The listing builds one solid part. Answer for the finished solid, in the listing's coordinates (mm). A direction names the side the tool comes from. Coordinates: 2 decimals unless noted, no trailing zeros. Loops run counter-clockwise (first coordinate to the right, second up) from the corner with the lowest first, then second, coordinate; pieces in that order, holes last. Notation, with made-up numbers: M -9,21 L 9,21 A6 cw 9,29 Z; hole C 41.5,89.25 d11. An arc over 180 degrees is marked long. Answer in a Markdown table with one row per item. Add a question column.
from build123d import *

# Parameters (mm, degrees)
SKETCH_1_W          = 166
SKETCH_1_H          = 70
EXTRUDE_1_DEPTH     = 3
SKETCH_2_W          = 3
SKETCH_2_H          = 20
CUT_EXTRUDE_1_DEPTH = 91.1276872
SKETCH_3_R          = 1.5
CUT_EXTRUDE_2_DEPTH = 91.1276872
SKETCH_4_R          = 1
CUT_EXTRUDE_3_DEPTH = 91.1276872
FILLET_1_R          = 1
SKETCH_5_R          = 22.5
CUT_EXTRUDE_4_DEPTH = 91.1276872
SKETCH_6_R          = 2.5
CUT_EXTRUDE_5_DEPTH = 91.1276872
FILLET_2_R          = 10
SKETCH_7_W          = 30
SKETCH_7_H          = 10
EXTRUDE_2_DEPTH     = 3
FILLET_START        = -1
FILLET_3_DEPTH      = 5
FILLET_3_2_DEPTH    = 3
SKETCH_8_R          = 1.5
CUT_EXTRUDE_6_DEPTH = 95.461632423
SKETCH_9_R          = 1.5
CUT_EXTRUDE_7_DEPTH = 95.461632423


with BuildPart() as part:
    # 草图1 → 凸台-拉伸1 (new body)
    with BuildSketch(Plane.XY):
        Rectangle(SKETCH_1_W, SKETCH_1_H)
    extrude(amount=EXTRUDE_1_DEPTH)

    # 草图2 → 切除-拉伸1 (cut, through all)
    with BuildSketch(Plane.XY.offset(3)):
        with Locations((-81.5, 0)):
            Rectangle(SKETCH_2_W, SKETCH_2_H)
    extrude(amount=-CUT_EXTRUDE_1_DEPTH, mode=Mode.SUBTRACT)

    # 草图3 → 切除-拉伸2 (cut, through all)
    with BuildSketch(Plane.XY.offset(3)):
        with Locations((-77, 27)):
            Circle(SKETCH_3_R)
        with Locations((-77, 17)):
            Circle(SKETCH_3_R)
        with Locations(Location((-77, -17, 0), (0, 0, 180))):
            Circle(SKETCH_3_R)
        with Locations(Location((-77, -27, 0), (0, 0, 180))):
            Circle(SKETCH_3_R)
    extrude(amount=-CUT_EXTRUDE_2_DEPTH, mode=Mode.SUBTRACT)

    # 草图4 → 切除-拉伸3 (cut, through all)
    with BuildSketch(Plane.XY.offset(3)):
        with Locations((-10, 22.6)):
            Circle(SKETCH_4_R)
        with Locations((8, 22.6)):
            Circle(SKETCH_4_R)
        with Locations(Location((8, -22.6, 0), (0, 0, 180))):
            Circle(SKETCH_4_R)
        with Locations(Location((-10, -22.6, 0), (0, 0, 180))):
            Circle(SKETCH_4_R)
    extrude(amount=-CUT_EXTRUDE_3_DEPTH, mode=Mode.SUBTRACT)

    # 圆角1
    fillet_1_edges = [part.edges().sort_by_distance(p)[0] for p in [
        (-83, -10, 1.5),
        (-83, 10, 1.5),
        (-83, -35, 1.5),
        (-83, 35, 1.5),
    ]]
    fillet(fillet_1_edges, radius=FILLET_1_R)

    # 草图5 → 切除-拉伸4 (cut, through all)
    with BuildSketch(Plane.XY.offset(3)):
        with Locations((38, 0)):
            Circle(SKETCH_5_R)
    extrude(amount=-CUT_EXTRUDE_4_DEPTH, mode=Mode.SUBTRACT)

    # 草图6 → 切除-拉伸5 (cut, through all)
    with BuildSketch(Plane.XY.offset(3)):
        with Locations((75, 27)):
            Circle(SKETCH_6_R)
        with Locations((-25, 27)):
            Circle(SKETCH_6_R)
        with Locations(Location((75, -27, 0), (0, 0, 180))):
            Circle(SKETCH_6_R)
        with Locations(Location((-25, -27, 0), (0, 0, 180))):
            Circle(SKETCH_6_R)
    extrude(amount=-CUT_EXTRUDE_5_DEPTH, mode=Mode.SUBTRACT)

    # 圆角2
    fillet_2_edges = [part.edges().sort_by_distance(p)[0] for p in [
        (83, -35, 1.5),
        (83, 35, 1.5),
    ]]
    fillet(fillet_2_edges, radius=FILLET_2_R)

    # 草图7 → 凸台-拉伸2 (add)
    with BuildSketch(Plane.XY.offset(3)):
        with Locations((28, 40)):
            Rectangle(SKETCH_7_W, SKETCH_7_H)
        with Locations((28, -40)):
            Rectangle(SKETCH_7_W, SKETCH_7_H)
    extrude(amount=-EXTRUDE_2_DEPTH)

    # 圆角3: read off the stored shape, not the designer's step
    # 圆角3 outline → 圆角3 (cut)
    with BuildSketch(Plane.XY.offset(FILLET_START)):
        with BuildLine():
            Line((13, -45), (18, -45))
            ThreePointArc((18, -45), (14.464466094, -43.535533906), (13, -40))
            Line((13, -40), (13, -45))
        make_face()
        with BuildLine():
            ThreePointArc((43, -40), (41.535533906, -43.535533906), (38, -45))
            Line((38, -45), (43, -45))
            Line((43, -45), (43, -40))
        make_face()
        with BuildLine():
            Line((43, 45), (38, 45))
            ThreePointArc((38, 45), (41.535533906, 43.535533906), (43, 40))
            Line((43, 40), (43, 45))
        make_face()
        with BuildLine():
            ThreePointArc((13, 40), (14.464466094, 43.535533906), (18, 45))
            Line((18, 45), (13, 45))
            Line((13, 45), (13, 40))
        make_face()
    extrude(amount=FILLET_3_DEPTH, mode=Mode.SUBTRACT)

    # Fillet 3 2 outline → Fillet 3 2 (add)
    with BuildSketch(Plane.XY):
        with BuildLine():
            Line((43, -35), (43, -40))
            ThreePointArc((43, -40), (44.464466094, -36.464466094), (48, -35))
            Line((48, -35), (43, -35))
        make_face()
        with BuildLine():
            ThreePointArc((8, -35), (11.535533906, -36.464466094), (13, -40))
            Line((13, -40), (13, -35))
            Line((13, -35), (8, -35))
        make_face()
        with BuildLine():
            Line((13, 35), (13, 40))
            ThreePointArc((13, 40), (11.535533906, 36.464466094), (8, 35))
            Line((8, 35), (13, 35))
        make_face()
        with BuildLine():
            ThreePointArc((48, 35), (44.464466094, 36.464466094), (43, 40))
            Line((43, 40), (43, 35))
            Line((43, 35), (48, 35))
        make_face()
    extrude(amount=FILLET_3_2_DEPTH)

    # 草图8 → 切除-拉伸6 (cut, through all)
    with BuildSketch(Plane(origin=(0, 0, 0), x_dir=(-1, 0, 0), z_dir=(0, 0, -1))):
        with Locations((-78, 0)):
            Circle(SKETCH_8_R)
    extrude(amount=-CUT_EXTRUDE_6_DEPTH, mode=Mode.SUBTRACT)

    # 草图9 → 切除-拉伸7 (cut, through all)
    with BuildSketch(Plane(origin=(0, 0, 0), x_dir=(-1, 0, 0), z_dir=(0, 0, -1))):
        with Locations((-29, 40)):
            Circle(SKETCH_9_R)
        with Locations(Location((-29, -40, 0), (0, 0, 180))):
            Circle(SKETCH_9_R)
    extrude(amount=-CUT_EXTRUDE_7_DEPTH, mode=Mode.SUBTRACT)


solid = part.part
(1) A cutting plane is placed at B-B (x = 20.5). Give the vertices of the cut face in (y, z), plus the area to 3 significant figures.
(2) A cutting plane is placed at D-D (x = 1). Give the vertices of the cut face in (y, z), plus the area to 3 significant figures.
(3) Each of these flat-tipped pins is pushed along its axis until it touches: pin 1 (3 mm diameter, centred on x = 75, y = 27, fed in from -Z); pin 2 (1.5 mm diameter, centred on y = -1, z = 2, fed in from -X); pin 3 (1.6 mm diameter, centred on x = -81, z = 1, fed in from -Y). Where does it stop, or does it pass through?
(4) Straight lines are drawn through the part: line 1 (Y direction, x = -77, z = 2.3); line 2 (X direction, y = -22.6, z = 1.6); line 3 (Y direction, x = -25, z = 2.3). For each, find the intervals that lie inside material, in ascending order.
(5) A cutting plane is placed at A-A (x = -25). Give the vertices of the cut face in (y, z).
(6) For faces 1 (the face through (-38, -35, 1)), 2 (the face through (-80, 0, 2)), 3 (the face through (-1, 1, 0)), 4 (the face through (-38, 35, 1)), 5 (the face through (27.8, -39.1, 1.5)), determine the directions among +Z, -Z, +X, -X, +Y, -Y from which every point of the face is accessible in a straight line to the end or side of a thin tool.
(7) A cutting plane is placed at C-C (z = 1.1). State how many separate pieces and enclosed holes the cut face has, plus the area to 3 significant figures.
Solved:
| question | item | result |
|---|---|---|
| 1 | outline | M -45,0 L -14.14,0 L -14.14,3 L -45,3 Z; M 14.14,0 L 45,0 L 45,3 L 14.14,3 Z |
| 1 | area | 185 mm² |
| 2 | outline | M -35,0 L 35,0 L 35,3 L -35,3 Z |
| 2 | area | 210 mm² |
| 3 | pin 1 | passes through |
| 3 | pin 2 | stops at x = -80 |
| 3 | pin 3 | stops at y = -35 |
| 4 | line 1 | y = -35 to -28.5, -25.5 to -18.5, -15.5 to 15.5, 18.5 to 25.5, 28.5 to 35 |
| 4 | line 2 | x = -83 to -11, -9 to 7, 9 to 83 |
| 4 | line 3 | y = -35 to -29.5, -24.5 to 24.5, 29.5 to 35 |
| 5 | outline | M -35,0 L -29.5,0 L -29.5,3 L -35,3 Z; M -24.5,0 L 24.5,0 L 24.5,3 L -24.5,3 Z; M 29.5,0 L 35,0 L 35,3 L 29.5,3 Z |
| 6 | face 1 | +Z, -Z, -X, -Y |
| 6 | face 2 | +Z, -Z, -X |
| 6 | face 3 | -Z, +X, -X, +Y, -Y |
| 6 | face 4 | +Z, -Z, -X, +Y |
| 6 | face 5 | +Z, -Z |
| 7 | separate pieces | 1 |
| 7 | enclosed holes | 16 |
| 7 | area | 10,400 mm² |
